Can you work these out from the model? Positions are in its coordinate system, mm. A direction names the side the tool comes from. Give positions to 0.01 mm unless a question says otherwise; leave off trailing zeros. Order: outer loops, then holes, each group sorted by start corner. A loop starts at its lowest first (then second) coordinate and runs counter-clockwise, first axis right, second up. Notation, with made-up numbers: M 50.5,70 L 70.5,70 A25 cw 70.5,94 Z; hole C 41.25,61.25 d9. An arc over 180 degrees is marked long. Answer as a JSON object with one key per item and string values.
```python
from build123d import *

# Parameters (mm, degrees)
SKETCH1_W           = 6
SKETCH1_H           = 80
SKETCH1_W_2         = 120
SKETCH1_H_2         = 6
BOSS_EXTRUDE1_DEPTH = 100
CUT_EXTRUDE1_DEPTH  = 120


with BuildPart() as part:
    # Sketch1 → Boss-Extrude1 (new body)
    with BuildSketch(Plane(origin=(0, 0, 0), x_dir=(1, 0, 0), z_dir=(0, 1, 0))):
        with Locations((57, -43)):
            Rectangle(SKETCH1_W, SKETCH1_H)
        Rectangle(SKETCH1_W_2, SKETCH1_H_2)
        with Locations((-57, -43)):
            Rectangle(SKETCH1_W, SKETCH1_H)
    extrude(amount=BOSS_EXTRUDE1_DEPTH)

    # Sketch2 → Cut-Extrude1 (cut)
    with BuildSketch(Plane.ZY.offset(60)):
        Polygon((83, 0), (-3, 100), (83, 100), align=None)
    extrude(amount=-CUT_EXTRUDE1_DEPTH, mode=Mode.SUBTRACT)


solid = part.part
```
1) I want a section at A-A on z = 67. Write out the boundary of the cut face in (x, y).
Results found:
{"outline": "M -60,0 L -54,0 L -54,18.6 L -60,18.6 Z; M 54,0 L 60,0 L 60,18.6 L 54,18.6 Z"}
2) For faces 4 (the face through (-54, 25, 26)), 5 (the face through (-0.28, 94.21, 1.98)), which set-ups out of +Z, -Z, +X, -X, +Y, -Y let a thin tool reach every point of the face, with its end or its side?
Results found:
{"face 4": "+Z, +Y, -Y", "face 5": "+Z, +X, -X, +Y"}
3) I want a section at C-C on x = 13.5. Write out the boundary of the cut face in (y, z), and give its area (3 significant figures).
Results found:
{"outline": "M 0,-3 L 100,-3 L 93.02,3 L 0,3 Z", "area": "579 mm²"}
4) Thinking about a two-plate mould opening in X: for faces 1 (the face through (-1, 46, 3)), 2 (the face through (-5, 0, 2)), 3 (the face through (60, 27, 21)), which applies, pulls with the +X half, pulls with the -X half, needs draft (parallel to the pull), parting line crosses it, or undercut?
Results found:
{"face 1": "undercut", "face 2": "needs draft", "face 3": "pulls with the +X half"}
5) I want a section at D-D on z = 31. Write out the boundary of the cut face in (x, y).
Results found:
{"outline": "M -60,0 L -54,0 L -54,60.47 L -60,60.47 Z; M 54,0 L 60,0 L 60,60.47 L 54,60.47 Z"}
6) I'm going to push a flat-ended pin straight in: pin 1 Ø2 at (x, y) = (42, 73) entering from +Z. Where does the tip first touch, or does it pass through?
Results found:
{"pin 1": "stops at z = 3"}
7) I need wall thicknesses on L1, parallel to X at y = 25, z = 47.5; L2, parallel to Z at x = 4, y = 80; L3, parallel to Z at x = 6, y = 94.5. Which ranges of each line are inside material? Lowest first, please.
Results found:
{"L1": "x = -60 to -54, 54 to 60", "L2": "z = -3 to 3", "L3": "z = -3 to 1.73"}
8) I want a section at B-B on y = 70. Write out the boundary of the cut face in (x, z).
Results found:
{"outline": "M -60,-3 L 60,-3 L 60,22.8 L 54,22.8 L 54,3 L -54,3 L -54,22.8 L -60,22.8 Z"}
